from build123d import *

# Parameters (mm, degrees)
SKETCH_1_R                = 22
EXTRUDE_1_DEPTH           = 15
SKETCH_6_R                = 30
EXTRUDE_2_DEPTH           = 6
CUT_EXTRUDE_1_DEPTH       = 46
CUT_EXTRUDE_1_DEPTH_BACK  = 46
SKETCH_2_R                = 2
SKETCH_3_R                = 10
CUT_EXTRUDE_2_DEPTH       = 46
HOLE_WIZARD_1_D           = 4.5
HOLE_WIZARD_1_CBORE_D     = 8
HOLE_WIZARD_1_CBORE_DEPTH = 4.6
HOLE_WIZARD_M4_1_D        = 3.3


with BuildPart() as part:
    # 草图1 → 凸台-拉伸1 (new body)
    with BuildSketch(Plane.XY):
        Circle(SKETCH_1_R)
    extrude(amount=EXTRUDE_1_DEPTH)

    # 草图6 → 凸台-拉伸2 (add)
    with BuildSketch(Plane(origin=(0, 0, 0), x_dir=(-1, 0, 0), z_dir=(0, 0, -1))):
        Circle(SKETCH_6_R)
    extrude(amount=-EXTRUDE_2_DEPTH)

    # 草图2 → 切除-拉伸1 (cut, two sides: drawn at the far end of the back side and taken through both)
    with BuildSketch(Plane.XY.offset(15).offset(-CUT_EXTRUDE_1_DEPTH_BACK)):
        with Locations((-12.340862004, 7.125)):
            Circle(SKETCH_2_R)
        with Locations((12.340862004, 7.125)):
            Circle(SKETCH_2_R)
        with Locations((0, -14.25)):
            Circle(SKETCH_2_R)
    extrude(amount=CUT_EXTRUDE_1_DEPTH + CUT_EXTRUDE_1_DEPTH_BACK, mode=Mode.SUBTRACT)

    # 草图3 → 切除-拉伸2 (cut, through all)
    with BuildSketch(Plane(origin=(0, 0, 0), x_dir=(-1, 0, 0), z_dir=(0, 0, -1))):
        Circle(SKETCH_3_R)
    extrude(amount=-CUT_EXTRUDE_2_DEPTH, mode=Mode.SUBTRACT)

    # 打孔尺寸(%根据)内六角圆柱头螺钉的类型1 (through all)
    with Locations(Plane(origin=(12.990381057, -7.5, 0), x_dir=(-1, 0, 0), z_dir=(0, 0, -1))):
        with Locations((0, 0), (25.980762114, 0), (12.990381057, 22.5)):
            CounterBoreHole(HOLE_WIZARD_1_D / 2, HOLE_WIZARD_1_CBORE_D / 2, HOLE_WIZARD_1_CBORE_DEPTH)

    # M4 螺纹孔1 (through all)
    with Locations(Plane(origin=(25, 0, 0), x_dir=(-1, 0, 0), z_dir=(0, 0, -1))):
        with Locations((0, 0), (12.5, 21.650635095), (37.5, 21.650635095), (50, 0), (37.5, -21.650635095), (12.5, -21.650635095)):
            Hole(HOLE_WIZARD_M4_1_D / 2)


solid = part.part
Can you work these out from the model? Positions are in its coordinate system, mm. A direction names the side the tool comes from. Round coordinates to 2 decimals unless told otherwise and drop trailing zeros. Order: outer loops, then holes, each group sorted by start corner. A loop starts at its lowest first (then second) coordinate and runs counter-clockwise, first axis right, second up. Notation, with made-up numbers: (25, 29.5) - (38, 29.5) arc R15 cw to (38, 36.5) - close; hole circle Ø2 at (-16, 78.5). An arc over 180 degrees is marked (long way). Answer in a Markdown table with one row per item.
(1) Suppose I cut it at D-D, the plane y = 13.5. Please give me the cut outline in (x, z), plus the area to 3 significant figures.
From the geometry:
| item | result |
|---|---|
| outline | (-26.79, 0) - (-3.71, 0) - (-3.71, 4.6) - (-1.68, 4.6) - (-1.68, 15) - (-17.37, 15) - (-17.37, 6) - (-26.79, 6) - close; (1.68, 4.6) - (3.71, 4.6) - (3.71, 0) - (26.79, 0) - (26.79, 6) - (17.37, 6) - (17.37, 15) - (1.68, 15) - close |
| area | 565 mm2 |
(2) Please list where these lines run through material, in increasing order: L1, parallel to Y at x = 0, z = 10.75; L2, parallel to X at y = -8, z = 5.5; L3, parallel to Y at x = 1.5, z = 3.75. Write a range as from..to.
From the geometry:
| item | result |
|---|---|
| L1 | y = -22..-16.25, -12.25..-10, 10..12.75, 17.25..22 |
| L2 | x = -28.91..-15.18, -10.8..-6, 6..10.8, 15.18..28.91 |
| L3 | y = -29.96..-15.57, -12.93..-9.89, 9.89..11.29, 18.71..29.96 |
(3) Suppose I cut it at C-C, the plane z = 12.25. Please give me the cut outline in (x, y) (3 decimals).
From the geometry:
| item | result |
|---|---|
| outline | circle Ø44 at (0, 0); hole circle Ø4.5 at (-12.99, -7.5); hole circle Ø4 at (-12.341, 7.125); hole circle Ø20 at (0, 0); hole circle Ø4.5 at (0, 15); hole circle Ø4 at (0, -14.25); hole circle Ø4 at (12.341, 7.125); hole circle Ø4.5 at (12.99, -7.5) |
(4) If we mould it in two halves opening along Y, with no side actions, what happens to faces 3 (the face through (-4.769, -21.477, 10.437)), 4 (the face through (-13.81, 8.48, 7.39)), 5 (the face through (2.4, 22.4, 6))? For each: released by +Y, released by -Y, zero draft, split by the parting line, or undercut.
From the geometry:
| item | result |
|---|---|
| face 3 | split by the parting line |
| face 4 | undercut |
| face 5 | zero draft |
(5) For P1, Ø2, axis at x = 7.5, y = -17, coming from the -Z side; P2, Ø6.5, axis at x = 12.99, y = -7.5, coming from the -Z side; P3, Ø5, axis at y = 21.5, z = 13, coming from the -X side; P4, Ø8, axis at x = 18.5, z = 3, coming from the +Y side, each with a flat end and sliding along its axis, tell me the tip position at first contact or that it passes through.
From the geometry:
| item | result |
|---|---|
| P1 | stops at z = 0 |
| P2 | stops at z = 4.6 |
| P3 | stops at x = -11.09 |
| P4 | stops at y = 26.26 |
(6) Suppose I cut it at B-B, the plane y = 0. Please give me the cut outline in (x, z).
From the geometry:
| item | result |
|---|---|
| outline | (-30, 0) - (-26.65, 0) - (-26.65, 6) - (-30, 6) - close; (-23.35, 0) - (-10, 0) - (-10, 15) - (-22, 15) - (-22, 6) - (-23.35, 6) - close; (10, 0) - (23.35, 0) - (23.35, 6) - (22, 6) - (22, 15) - (10, 15) - close; (26.65, 0) - (30, 0) - (30, 6) - (26.65, 6) - close |
(7) Suppose I cut it at A-A, the plane x = 0. Please give me the cut outline in (y, z).
From the geometry:
| item | result |
|---|---|
| outline | (-30, 0) - (-16.25, 0) - (-16.25, 15) - (-22, 15) - (-22, 6) - (-30, 6) - close; (-12.25, 0) - (-10, 0) - (-10, 15) - (-12.25, 15) - close; (10, 0) - (11, 0) - (11, 4.6) - (12.75, 4.6) - (12.75, 15) - (10, 15) - close; (17.25, 4.6) - (19, 4.6) - (19, 0) - (30, 0) - (30, 6) - (22, 6) - (22, 15) - (17.25, 15) - close |
(8) Which directions (+Z, -Z, +X, -X, +Y, -Y) give clear straight access to the entire face, cutting with the end or side of a thin tool? Please do faces 1 (the face through (5, -9, 15)), 2 (the face through (-15, -9, 4.6)).
From the geometry:
| item | result |
|---|---|
| face 1 | +Z, +X, -X, +Y, -Y |
| face 2 | -Z |
